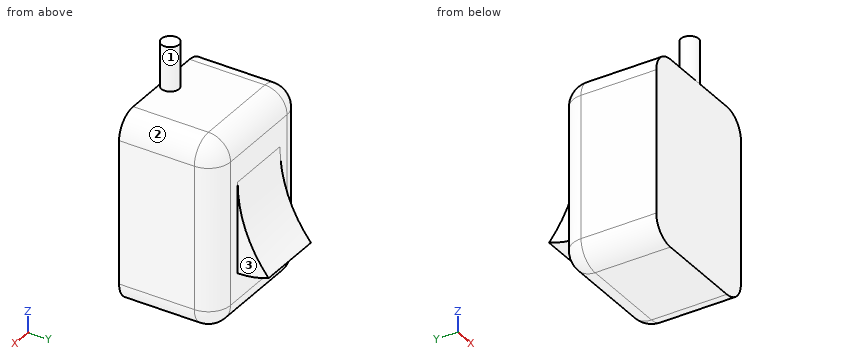
from build123d import *

# Parameters (mm, degrees)
SKETCH1_W           = 30
SKETCH1_H           = 42.3
BOSS_EXTRUDE1_DEPTH = 22
SKETCH2_R           = 2
BOSS_EXTRUDE2_DEPTH = 10
FILLET2_R           = 5
BOSS_EXTRUDE4_DEPTH = 30
CUT_EXTRUDE1_DEPTH  = 7.5
CUT_EXTRUDE2_START  = -7.5
CUT_EXTRUDE2_DEPTH  = 7.5


with BuildPart() as part:
    # Sketch1 → Boss-Extrude1 (new body)
    with BuildSketch(Plane(origin=(0, 0, 0), x_dir=(1, 0, 0), z_dir=(0, 1, 0))):
        with Locations((15, 21.15)):
            Rectangle(SKETCH1_W, SKETCH1_H)
    extrude(amount=BOSS_EXTRUDE1_DEPTH)

    # Sketch2 → Boss-Extrude2 (add)
    with BuildSketch(Plane.XY):
        with Locations(Location((15, 2, 0), (0, 0, 270))):
            Circle(SKETCH2_R)
    extrude(amount=BOSS_EXTRUDE2_DEPTH)

    # Fillet2
    fillet2_edges = [part.edges().sort_by_distance(p)[0] for p in [
        (30, 22, -21.15),
        (15, 22, -42.3),
        (0, 22, -21.15),
        (0, 11, -42.3),
        (30, 11, -42.3),
        (30, 11, 0),
        (0, 11, 0),
        (15, 22, 0),
    ]]
    fillet(fillet2_edges, radius=FILLET2_R)

    # Sketch5 → Boss-Extrude4 (add)
    with BuildSketch(Plane(origin=(0, 0, 0), x_dir=(0, 0, -1), z_dir=(1, 0, 0))):
        with BuildLine():
            Line((10.886815905, 22), (31.413184095, 22))
            ThreePointArc((31.413184095, 22), (31.094391882, 25.55669229), (30.14817809, 29))
            ThreePointArc((30.14817809, 29), (21.133767679, 23.804255316), (10.886815905, 22))
        make_face()
    extrude(amount=BOSS_EXTRUDE4_DEPTH)

    # Sketch6 → Cut-Extrude1 (cut)
    with BuildSketch(Plane.ZY):
        with BuildLine():
            Line((-10.886815905, 22), (-31.413184095, 22))
            ThreePointArc((-31.413184095, 22), (-31.094391882, 25.55669229), (-30.14817809, 29))
            ThreePointArc((-30.14817809, 29), (-21.133767679, 23.804255316), (-10.886815905, 22))
        make_face()
    extrude(amount=-CUT_EXTRUDE1_DEPTH, mode=Mode.SUBTRACT)

    # Sketch7 → Cut-Extrude2 (cut)
    with BuildSketch(Plane(origin=(30, 0, 0), x_dir=(0, 0, -1), z_dir=(1, 0, 0)).offset(CUT_EXTRUDE2_START)):
        with BuildLine():
            Line((10.886815905, 22), (31.413184095, 22))
            ThreePointArc((31.413184095, 22), (31.094391882, 25.55669229), (30.14817809, 29))
            ThreePointArc((30.14817809, 29), (21.133767679, 23.804255316), (10.886815905, 22))
        make_face()
    extrude(amount=CUT_EXTRUDE2_DEPTH, mode=Mode.SUBTRACT)


solid = part.part
Check sheet for the modelled part. Datum: model origin and axes. Units: mm. Face numbers are marked on the shaded views. A direction names the side the tool comes from. Round coordinates to 2 decimals unless told otherwise and drop trailing zeros. Order: outer loops, then holes, each group sorted by start corner. A loop starts at its lowest first (then second) coordinate and runs counter-clockwise, first axis right, second up.
Q1. Cross-section at D-D, the plane x = 23.25. Enter the section's corners in (y, z).
Filled sheet:
outline: (0, -42.3) - (17, -42.3) arc R5 ccw to (22, -37.3) - (22, -5) arc R5 ccw to (17, 0) - (0, 0) - close
Q2. Cross-section at B-B, the plane y = 2. Enter the section's corners in (x, z), plus the area to 3 significant figures.
Filled sheet:
outline: (0, -37.3) arc R5 ccw to (5, -42.3) - (25, -42.3) arc R5 ccw to (30, -37.3) - (30, -5) arc R5 ccw to (25, 0) - (17, 0) - (17, 10) - (13, 10) - (13, 0) - (5, 0) arc R5 ccw to (0, -5) - close
area: 1,290 mm2
Q3. Scan lines: L1, parallel to Y at x = 24.75, z = -24; L2, parallel to X at y = 27.75, z = -30; L3, parallel to Z at x = 20, y = 4.5. Record each from-to range of solid material in increasing order.
Filled sheet:
L1: y = 0 to 22
L2: x = 7.5 to 22.5
L3: z = -42.3 to 0
Q4. Set-up check for the marked faces 1, 2 and 3: record each of +Z, -Z, +X, -X, +Y, -Y from which the full face is reachable in a straight line by a thin tool's end or side.
Filled sheet:
face 1: +Z
face 2: +Z, +X, +Y, -Y
face 3: +Z, -Z, +X, +Y
Q5. Cross-section at A-A, the plane x = 19. Enter the section's corners in (y, z).
Filled sheet:
outline: (0, -42.3) - (17, -42.3) arc R5 ccw to (22, -37.3) - (22, -31.41) arc R20 ccw to (29, -30.15) arc R30 cw to (22, -10.89) - (22, -5) arc R5 ccw to (17, 0) - (0, 0) - close
Q6. Depth check by flat-ended pin: P1, Ø12, axis at x = 23, y = 7, coming from the +Z side; P2, Ø1, axis at x = 8.5, z = -17.5, coming from the +Y side; P3, Ø6, axis at x = 20, z = -20.5, coming from the +Y side; P4, Ø7.5, axis at y = 27, z = -17, coming from the -X side. Enter the tip coordinate at first touch or a pass-through.
Filled sheet:
P1: stops at z = 0
P2: stops at y = 22.86
P3: stops at y = 24.78
P4: passes through
Q7. Cross-section at C-C, the plane z = -24.5. Enter the section's corners in (x, y).
Filled sheet:
outline: (0, 0) - (30, 0) - (30, 17) arc R5 ccw to (25, 22) - (22.5, 22) - (22.5, 25.27) - (7.5, 25.27) - (7.5, 22) - (5, 22) arc R5 ccw to (0, 17) - close
